Geometry check sheet. Reference: the model listing, model coordinates, mm. A direction names the side the tool comes from. Coordinates: 2 decimals unless noted, no trailing zeros. Write each loop counter-clockwise with the first axis right and the second up, starting at its lowest first coordinate (ties: lowest second). Pieces come first, ordered by that corner, then holes. Notation, with made-up numbers: M 60.25,33.25 L 68.25,33.25 A6 ccw 68.25,40.25 Z; hole C -26,49.5 d9. An arc over 180 degrees is marked long. Put each result on its own line as item: value. Start each with the question number.
1) Scan lines: line 1 along X through (y, z) = (37.5, 3.2); line 2 along Y through (x, z) = (-117.5, 2.4); line 3 along X through (y, z) = (-9, 1.8). Record each from-to range of solid material in increasing order.
2) Cross-section at D-D on x = -143.5. Record the cut outline in (y, z).
3) Cross-section at C-C on y = 2. Record the cut outline in (x, z), plus the area to 3 significant figures.
4) Cross-section at A-A on y = 37.5. Record the cut outline in (x, z).
5) Gauge pin test, flat ends, axial feed: pin 1 (0.5 mm diameter, centred on x = -87, z = 1.5, fed in from +Y); pin 2 (1 mm diameter, centred on y = 19.5, z = 2, fed in from +X); pin 3 (1.5 mm diameter, centred on x = -113, z = 2.5, fed in from -Y); pin 4 (2.5 mm diameter, centred on x = -117.65, y = 27.805, fed in from -Z). Record the tip position at first contact, or that the pin passes through.
6) Mould release check, pull along Y, two halves, no side actions. Record for faces 4 (the flat face through (-63, -41.7, 2.5)), 5 (the flat face through (-109, 1, 0)), 6 (the flat face through (-62.883, 41.723, 2.465)), 7 (the cylindrical face through (-59.66, -35.98, 2.46)): released by +Y, released by -Y, zero draft, split by the parting line, or undercut.
7) Set-up check for faces 1 (the flat face through (-107, -41, 2)), 2 (the flat face through (-89, -28, 2)), 3 (the flat face through (-109, 41, 2)): record each of +Z, -Z, +X, -X, +Y, -Y from which the full face is reachable in a straight line by a thin tool's end or side.
8) Cross-section at B-B on x = -117.65. Record the cut outline in (y, z) (3 decimals).
from build123d import *

# Parameters (mm, degrees)
SKETCH111_W     = 80
SKETCH111_H     = 80
PAD042_DEPTH    = 5
SKETCH112_W     = 82
SKETCH112_H     = 82
PAD043_DEPTH    = 1
SKETCH114_R     = 3
SKETCH114_R_2   = 1.375
PAD045_DEPTH    = 4
SKETCH215_W     = 16
SKETCH215_H     = 3
PAD095_DEPTH    = 2
SKETCH216_R     = 2.25
POCKET088_DEPTH = 10
SKETCH217_W     = 10
SKETCH217_H     = 2
POCKET089_DEPTH = 5
SKETCH255_R     = 1.5
POCKET103_DEPTH = 5


with BuildPart() as part:
    # Sketch111 → Pad042 (new body)
    with BuildSketch(Plane.XY):
        with BuildLine():
            Line((-41.02059, 41), (40.97941, 41))
            Line((49.139632, 42.42542), (40.97941, 41))
            ThreePointArc((50.860368, 32.57458), (54.92542, 38.360368), (49.139632, 42.42542))
            Line((41, 30.852179), (50.860368, 32.57458))
            Line((41, 30.852179), (41, -30.847821))
            Line((50.86248, -32.574949), (41, -30.847821))
            ThreePointArc((49.13752, -42.425051), (54.925051, -38.36248), (50.86248, -32.574949))
            Line((41, -41), (49.13752, -42.425051))
            Line((41, -41), (-41, -41))
            Line((-49.13752, -42.425051), (-41, -41))
            ThreePointArc((-50.86248, -32.574949), (-54.925051, -38.36248), (-49.13752, -42.425051))
            Line((-50.86248, -32.574949), (-41, -30.847821))
            Line((-41, -30.847821), (-41, 30.843439))
            Line((-41, 30.843439), (-50.864603, 32.575321))
            ThreePointArc((-49.135397, 42.424679), (-54.924679, 38.364603), (-50.864603, 32.575321))
            Line((-41.02059, 41), (-49.135397, 42.424679))
        make_face()
        Rectangle(SKETCH111_W, SKETCH111_H, mode=Mode.SUBTRACT)
    extrude(amount=PAD042_DEPTH)

    # Sketch112 → Pad043 (join)
    with BuildSketch(Plane.XY):
        Rectangle(SKETCH112_W, SKETCH112_H)
    extrude(amount=PAD043_DEPTH)

    # Sketch114 → Pad045 (join)
    with BuildSketch(Plane.XY):
        with Locations((-28.95, 27.805)):
            Circle(SKETCH114_R)
        with Locations((-28.95, 27.805)):
            Circle(SKETCH114_R_2, mode=Mode.SUBTRACT)
        with Locations((-9.65, 27.805)):
            Circle(SKETCH114_R)
        with Locations((-9.65, 27.805)):
            Circle(SKETCH114_R_2, mode=Mode.SUBTRACT)
        with Locations((9.65, 27.805)):
            Circle(SKETCH114_R)
        with Locations((9.65, 27.805)):
            Circle(SKETCH114_R_2, mode=Mode.SUBTRACT)
        with Locations((28.95, 27.805)):
            Circle(SKETCH114_R)
        with Locations((28.95, 27.805)):
            Circle(SKETCH114_R_2, mode=Mode.SUBTRACT)
        with Locations((28.95, -27.805)):
            Circle(SKETCH114_R)
        with Locations((28.95, -27.805)):
            Circle(SKETCH114_R_2, mode=Mode.SUBTRACT)
        with Locations((9.65, -27.805)):
            Circle(SKETCH114_R)
        with Locations((9.65, -27.805)):
            Circle(SKETCH114_R_2, mode=Mode.SUBTRACT)
        with Locations((-9.65, -27.805)):
            Circle(SKETCH114_R)
        with Locations((-9.65, -27.805)):
            Circle(SKETCH114_R_2, mode=Mode.SUBTRACT)
        with Locations((-28.95, -27.805)):
            Circle(SKETCH114_R)
        with Locations((-28.95, -27.805)):
            Circle(SKETCH114_R_2, mode=Mode.SUBTRACT)
    extrude(amount=PAD045_DEPTH)

    # Sketch215 → Pad095 (join)
    with BuildSketch(Plane.XY):
        with Locations((-20, 28)):
            Rectangle(SKETCH215_W, SKETCH215_H)
        with Locations((20, 28)):
            Rectangle(SKETCH215_W, SKETCH215_H)
        with Locations((-20, -28)):
            Rectangle(SKETCH215_W, SKETCH215_H)
        with Locations((20, -28)):
            Rectangle(SKETCH215_W, SKETCH215_H)
        with Locations((0, 28)):
            Rectangle(SKETCH215_W, SKETCH215_H)
        with Locations((0, -28)):
            Rectangle(SKETCH215_W, SKETCH215_H)
    extrude(amount=PAD095_DEPTH)

    # Sketch216 → Pocket088 (cut)
    with BuildSketch(Plane.XY):
        with Locations((-50, 37.5)):
            Circle(SKETCH216_R)
        with Locations((50, 37.5)):
            Circle(SKETCH216_R)
        with Locations((50, -37.5)):
            Circle(SKETCH216_R)
        with Locations((-50, -37.5)):
            Circle(SKETCH216_R)
    extrude(amount=POCKET088_DEPTH, mode=Mode.SUBTRACT)

    # Sketch217 (on Face1 of Pocket088) → Pocket089 (cut)
    with BuildSketch(Plane(origin=(0, 41, 0), x_dir=(-1, 0, 0), z_dir=(0, 1, 0))):
        with Locations((0, 4)):
            Rectangle(SKETCH217_W, SKETCH217_H)
    extrude(amount=-POCKET089_DEPTH, mode=Mode.SUBTRACT)

    # Sketch255 → Pocket103 (cut, symmetric)
    with BuildSketch(Plane.XY):
        with Locations((-9.65, 27.805)):
            Circle(SKETCH255_R)
        with Locations((9.65, 27.805)):
            Circle(SKETCH255_R)
        with Locations((-9.65, -27.805)):
            Circle(SKETCH255_R)
        with Locations((9.65, -27.805)):
            Circle(SKETCH255_R)
        with Locations((-28.95, 27.805)):
            Circle(SKETCH255_R)
        with Locations((28.95, 27.805)):
            Circle(SKETCH255_R)
        with Locations((28.95, -27.805)):
            Circle(SKETCH255_R)
        with Locations((-28.95, -27.805)):
            Circle(SKETCH255_R)
    extrude(amount=POCKET103_DEPTH, both=True, mode=Mode.SUBTRACT)


with BuildPart() as part_1:
    # Body013 placement: moved
    add(part.part.moved(Location((-108, 0, 0))))


solid = part_1.part
Answer key:
1. line 1: x = -163 to -160.25, -155.75 to -148, -68 to -60.25, -55.75 to -53
1. line 2: y = -41 to -40, -30.8 to -29.3, -26.31 to -24.81, 24.81 to 26.31, 29.3 to 30.8, 40 to 41
1. line 3: x = -149 to -148, -68 to -67
2. outline: M -41,0 L 41,0 L 41,5 L 40,5 L 40,1 L -40,1 L -40,5 L -41,5 Z
3. outline: M -149,0 L -67,0 L -67,5 L -68,5 L -68,1 L -148,1 L -148,5 L -149,5 Z
3. area: 90.0 mm²
4. outline: M -163,0 L -160.25,0 L -160.25,5 L -163,5 Z; M -155.75,0 L -60.25,0 L -60.25,5 L -68,5 L -68,1 L -148,1 L -148,5 L -155.75,5 Z; M -55.75,0 L -53,0 L -53,5 L -55.75,5 Z
5. pin 1: stops at y = 41
5. pin 2: stops at x = -67
5. pin 3: stops at y = -41
5. pin 4: passes through
6. face 4: released by -Y
6. face 5: zero draft
6. face 6: released by +Y
6. face 7: undercut
7. face 1: +Z, -Z, -Y
7. face 2: +Z
7. face 3: +Z, -Z, +Y
8. outline: M -41,0 L -29.305,0 L -29.305,4 L -30.805,4 L -30.805,1 L -40,1 L -40,5 L -41,5 Z; M -26.305,0 L 26.305,0 L 26.305,4 L 24.805,4 L 24.805,1 L -24.805,1 L -24.805,4 L -26.305,4 Z; M 29.305,0 L 41,0 L 41,5 L 40,5 L 40,1 L 30.805,1 L 30.805,4 L 29.305,4 Z
